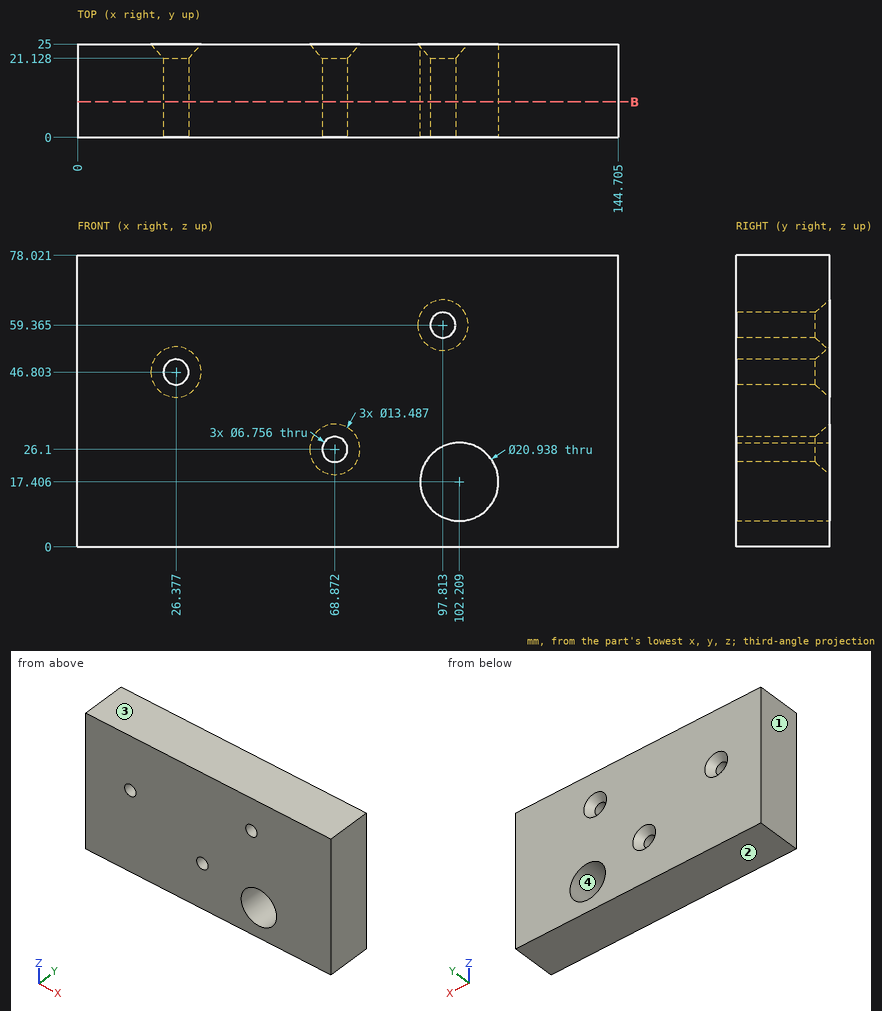
Can you work these out from the drawing? Everything is in mm from the part's minimum corner. Round coordinates to 2 decimals unless told otherwise and drop trailing zeros. Write each loop counter-clockwise with the first axis right and the second up, starting at its lowest first coordinate (ties: lowest second). Pieces come first, ordered by that corner, then holes.
1. If we mould it in two halves opening along Z, with no side actions, what happens to the marked faces 1, 2, 3 and 4? For each: released by +Z, released by -Z, zero draft, split by the parting line, or undercut.
2. Suppose I cut it at B-B (y = 9.5). List the corners of the cut face in (x, z) for me (1 decimal).
3. I need wall thicknesses on L1, parallel to Z at x = 95, y = 18 (1 decimal); L2, parallel to X at y = 9.75, z = 49.5 (1 decimal); L3, parallel to Z at x = 108, y = 3 (1 decimal). Which ranges of each line are inside material? Lowest first, please.
Answer sheet:
1. face 1: zero draft
1. face 2: released by -Z
1. face 3: released by +Z
1. face 4: undercut
2. outline: (0, 0) - (144.7, 0) - (144.7, 78) - (0, 78) - close; hole circle Ø6.8 at (26.4, 46.8); hole circle Ø6.8 at (68.9, 26.1); hole circle Ø20.9 at (102.2, 17.4); hole circle Ø6.8 at (97.8, 59.4)
3. L1: z = 0 to 9.8, 25 to 57.5, 61.2 to 78
3. L2: x = 0 to 24.3, 28.4 to 144.7
3. L3: z = 0 to 8.7, 26.1 to 78
